CAD build for the part. Positions are in the model's coordinates, mm. Coordinates: 2 decimals unless noted, no trailing zeros. Loops run counter-clockwise (first coordinate to the right, second up) from the corner with the lowest first, then second, coordinate; pieces in that order, holes last. Notation, with made-up numbers: (-10.5, -28.5) -> (21.5, -28.5) arc R17 cw to (21.5, -9.5) -> close; hole circle Ø9 at (71.5, 3.5). An arc over 180 degrees is marked (long way). Answer as a JSON object with one key per item and string values. Group by question number.
from build123d import *

# Parameters (mm, degrees)
SKETCH_1_R      = 2
SKETCH_1_R_2    = 4
EXTRUDE_1_DEPTH = 2


with BuildPart() as part:
    # 草图1 → 凸台-拉伸1 (new body)
    with BuildSketch(Plane.XY):
        with BuildLine():
            Line((-28.087756532, -25.18156201), (-37.652577321, -25.18156201))
            ThreePointArc((-37.652577321, -25.18156201), (-34.00481141, -29.821346246), (-29.792990581, -33.955878772))
            Line((-29.792990581, -33.955878772), (-6.740952381, -63.62952381))
            ThreePointArc((-6.740952381, -63.62952381), (0.259047619, -70.62952381), (7.259047619, -63.62952381))
            Line((7.259047619, -63.62952381), (12.392004443, -57.856149826))
            Line((12.392004443, -57.856149826), (12.193934029, -35.732918275))
            ThreePointArc((12.193934029, -35.732918275), (-9.496491359, -36.373039477), (-28.087756532, -25.18156201))
        make_face()
        with Locations((0.259047619, -41.62952381)):
            Circle(SKETCH_1_R, mode=Mode.SUBTRACT)
        with Locations((-29.792990581, -29.18156201)):
            Circle(SKETCH_1_R, mode=Mode.SUBTRACT)
        with Locations((0.259047619, -63.62952381)):
            Circle(SKETCH_1_R_2, mode=Mode.SUBTRACT)
    extrude(amount=EXTRUDE_1_DEPTH)


solid = part.part
Item 1: Pull direction X, two halves, no side cores. Call faces 1 (the cylindrical face through (-0.262, -59.664, 0.986)), 2 (the flat face through (-7, -48, 2)), 3 (the cylindrical face through (-34.06, -29.76, 0.99)), 4 (the flat face through (9.79, -60.78, 0.99)): +X half, -X half, draft (parallel to the pull), parting line (faces both ways), or undercut.
Item 2: Band-saw the part on C-C, the plane y = -30. List the corners of the cut face in (x, z).
Item 3: Band-saw the part on A-A, the plane y = -62.5. List the corners of the cut face in (x, z), and give its area (3 significant figures).
Item 4: Band-saw the part on D-D, the plane x = -21. List the corners of the cut face in (y, z), and give its area (3 significant figures).
Item 5: Band-saw the part on B-B, the plane z = 0.75. List the corners of the cut face in (x, y), and give its area (3 significant figures).
Item 6: Drill centre lines: L1, parallel to Y at x = -1, z = 1.95; L2, parallel to X at y = -30.5, z = 1.8; L3, parallel to X at y = -29, z = 0.15. Where is each one in solid material? Low to high.
Reply:
{
 "1": {"face 1": "undercut", "face 2": "draft", "face 3": "-X half", "face 4": "+X half"},
 "2": {"outline": "(-33.84, 0) -> (-31.62, 0) -> (-31.62, 2) -> (-33.84, 2) -> close; (-27.97, 0) -> (-22.75, 0) -> (-22.75, 2) -> (-27.97, 2) -> close"},
 "3": {"outline": "(-7.62, 0) -> (-3.58, 0) -> (-3.58, 2) -> (-7.62, 2) -> close; (4.1, 0) -> (8.26, 0) -> (8.26, 2) -> (4.1, 2) -> close", "area": "16.4 mm²"},
 "4": {"outline": "(-45.27, 0) -> (-31.23, 0) -> (-31.23, 2) -> (-45.27, 2) -> close", "area": "28.1 mm²"},
 "5": {"outline": "(-37.65, -25.18) arc R46 ccw to (-29.79, -33.96) -> (-6.74, -63.63) arc R7 ccw to (7.26, -63.63) -> (12.39, -57.86) -> (12.19, -35.73) arc R38.5 cw to (-28.09, -25.18) -> close; hole circle Ø4 at (-29.79, -29.18); hole circle Ø8 at (0.26, -63.63); hole circle Ø4 at (0.26, -41.63)", "area": "915 mm²"},
 "6": {"L1": "-70.52 to -67.43, -59.83 to -43.18, -40.08 to -37.61", "L2": "-33.38 to -31.3, -28.29 to -22.06", "L3": "-34.72 to -31.78, -27.8 to -24.03"}
}
